from build123d import *

# Parameters (mm, degrees)
SKETCH1_R           = 17
BOSS_EXTRUDE1_DEPTH = 6
BOSS_EXTRUDE1_TAPER = 5
SKETCH2_R           = 15.5
BOSS_EXTRUDE2_DEPTH = 12
BOSS_EXTRUDE2_TAPER = 5
SKETCH3_R           = 3.05
CUT_EXTRUDE1_DEPTH  = 17
FILLET1_R           = 1
FILLET2_R           = 0.5
SKETCH8_R           = 4.5
CUT_EXTRUDE6_DEPTH  = 8
FILLET3_R           = 0.5


with BuildPart() as part:
    # Sketch1 → Boss-Extrude1 (new body)
    with BuildSketch(Plane(origin=(0, 0, 0), x_dir=(1, 0, 0), z_dir=(0, 1, 0))):
        Circle(SKETCH1_R)
    extrude(amount=BOSS_EXTRUDE1_DEPTH, taper=BOSS_EXTRUDE1_TAPER)

    # Sketch2 → Boss-Extrude2 (add)
    with BuildSketch(Plane(origin=(0, 6, 0), x_dir=(1, 0, 0), z_dir=(0, 1, 0))):
        Circle(SKETCH2_R)
    extrude(amount=BOSS_EXTRUDE2_DEPTH, taper=BOSS_EXTRUDE2_TAPER)

    # Sketch3 → Cut-Extrude1 (cut)
    with BuildSketch(Plane.XZ):
        with Locations(Location((0, 0, 0), (0, 0, 270))):
            Circle(SKETCH3_R)
    extrude(amount=-CUT_EXTRUDE1_DEPTH, mode=Mode.SUBTRACT)

    # Fillet1
    fillet1_edges = [part.edges().sort_by_distance(p)[0] for p in [
        (-14.450136038, 18, 0),
    ]]
    fillet(fillet1_edges, radius=FILLET1_R)

    # Fillet2
    fillet2_edges = [part.edges().sort_by_distance(p)[0] for p in [
        (-16.475068019, 6, 0),
    ]]
    fillet(fillet2_edges, radius=FILLET2_R)

    # Sketch8 → Cut-Extrude6 (cut)
    with BuildSketch(Plane.XZ):
        with Locations(Location((0, 0, 0), (0, 0, 270))):
            Circle(SKETCH8_R)
    extrude(amount=-CUT_EXTRUDE6_DEPTH, mode=Mode.SUBTRACT)

    # Fillet3
    fillet3_edges = [part.edges().sort_by_distance(p)[0] for p in [
        (-17, 0, 0),
    ]]
    fillet(fillet3_edges, radius=FILLET3_R)


solid = part.part
For this review, take the finished solid that the model builds, in its own axes (mm). A direction names the side the tool comes from. Give positions to 0.01 mm unless a question says otherwise; leave off trailing zeros. Loops run counter-clockwise (first coordinate to the right, second up) from the corner with the lowest first, then second, coordinate; pieces in that order, holes last. Notation, with made-up numbers: M -10.75,41.25 L 35.25,41.25 A23 cw 35.25,57.25 Z; hole C -5,-36.75 d10. An arc over 180 degrees is marked long. Answer as a JSON object with one key per item and string values. Group by question number.
Q1. Add section C-C on y = 15.25. Give the boundary of the cut face in (x, z).
Q2. For probe 1 along X at (y, z) = (2.5, 3); probe 2 along Y at (x, z) = (-2.5, -1); probe 3 along X at (y, z) = (13.75, -11), list the stretches that pass through material, from the lowest coordinate up. Write a range as [from, to].
Q3. Mouldability with a two-part tool opening along X and no side actions: class faces 3 (the conical face through (-3.6, 4.75, 16.19)), 4 (the cylindrical face through (1.352, 3.944, -4.292)), 5 (the flat face through (0, 18, 0)) as +X half, -X half, draft (parallel to the pull), parting line (faces both ways), or undercut.
Q4. Add section B-B on y = 12. Give the boundary of the cut face in (x, z), and give its area (3 significant figures).
Q5. Insertion check: P1, Ø2, axis at x = -8, y = 2, coming from the -Z side; P2, Ø3, axis at x = 0.5, z = 0, coming from the -Y side; P3, Ø8, axis at x = 0, z = 0, coming from the -Y side. Each pin has a flat end and moves straight along its axis. Give the tip position at first contact, or say it passes through.
Q6. Add section A-A on x = 0. Give the boundary of the cut face in (y, z) (3 decimals).
Q7. Tool access review of faces 1 (the flat face through (3.4, 0, 3.4)), 2 (the cylindrical face through (-1.856, 12.437, 2.42)): name each direction out of +Z, -Z, +X, -X, +Y, -Y from which nothing blocks a thin tool from reaching the whole face with its end or side.
Checked values:
{
 "1": {"outline": "C 0,0 d29.38; hole C 0,0 d6.1"},
 "2": {"probe 1": "[-16.51, -3.35], [3.35, 16.51]", "probe 2": "[17, 18]", "probe 3": "[-9.93, 9.93]"},
 "3": {"face 3": "parting line", "face 4": "undercut", "face 5": "draft"},
 "4": {"outline": "C 0,0 d29.95; hole C 0,0 d6.1", "area": "675 mm²"},
 "5": {"P1": "z = -15.31", "P2": "y = 17", "P3": "y = 8"},
 "6": {"outline": "M 0,-16.454 A0.5 ccw 0.544,-16.952 L 5.544,-16.515 A0.5 ccw 6,-16.017 L 6,-15.5 L 17.087,-14.53 A1 ccw 18,-13.534 L 18,13.534 A1 ccw 17.087,14.53 L 6,15.5 L 6,16.017 A0.5 ccw 5.544,16.515 L 0.544,16.952 A0.5 ccw 0,16.454 L 0,4.5 L 8,4.5 L 8,3.05 L 17,3.05 L 17,-3.05 L 8,-3.05 L 8,-4.5 L 0,-4.5 Z"},
 "7": {"face 1": "+Z, -Z, +X, -X, -Y", "face 2": "-Y"}
}
